The listing builds one solid part. Answer for the finished solid, in the listing's coordinates (mm). A direction names the side the tool comes from. Give positions to 0.01 mm unless a question says otherwise; leave off trailing zeros. Loops run counter-clockwise (first coordinate to the right, second up) from the corner with the lowest first, then second, coordinate; pieces in that order, holes last. Notation, with made-up numbers: (20.5, 69) - (44.5, 69) arc R24 cw to (44.5, 105) - close; hole circle Ø1 at (80, 6.5). An arc over 180 degrees is marked (long way). Write each question's results on one line, items separated by ' | '.
Autodesk Inventor part; units mm, degrees
ref_plane "YZ Plane" through (0, 0, 0) normal (1, 0, 0) x (0, 1, 0)
ref_plane "XZ Plane" through (0, 0, 0) normal (0, 1, 0) x (-1, 0, 0)
ref_plane "XY Plane" through (0, 0, 0) normal (0, 0, 1) x (1, 0, 0)
sketch "Skizze1" plane through (0, 0, 0) normal (0, 0, 1) x (1, 0, 0)
  line L0 (-20, -3.5) -> (20, -3.5)
  line L1 (20, -3.5) -> (20, 3.5)
  line L2 (20, 3.5) -> (-20, 3.5)
  line L3 (-20, 3.5) -> (-20, -3.5)
  line L4 (-20, -3.5) -> (20, 3.5) construction
  line L5 (20, -3.5) -> (-20, 3.5) construction
  line L6 (3.5, -20) -> (-3.5, -20)
  line L7 (-3.5, -20) -> (-3.5, 20)
  line L8 (-3.5, 20) -> (3.5, 20)
  line L9 (3.5, 20) -> (3.5, -20)
  line L10 (3.5, -20) -> (-3.5, 20) construction
  line L11 (-3.5, -20) -> (3.5, 20) construction
  point P0 (0, 0)
  dimension "d0" = 7
  dimension "d1" = 40
extrude "Extrusion1" add sketch "Skizze1" along normal blind 1.5
fillet "Rundung1" radius 3.5 8 edges at (3.5, 20, 0.75) (-3.5, 20, 0.75) (20, 3.5, 0.75) (20, -3.5, 0.75) (3.5, -20, 0.75) (-3.5, -20, 0.75) (-20, -3.5, 0.75) (-20, 3.5, 0.75)
fillet "Rundung2" radius 6 4 edges at (3.5, 3.5, 0.75) (-3.5, 3.5, 0.75) (-3.5, -3.5, 0.75) (3.5, -3.5, 0.75)
sketch "Skizze2" plane through (0, 0, 1.5) normal (0, 0, 1) x (1, 0, 0)
  circle A0 centre (0, 0) radius 5
  circle A1 centre (16.5, 0) radius 1.6
  circle A2 centre (-16.5, 0) radius 1.6
  circle A3 centre (0, 16.5) radius 1.6
  circle A4 centre (0, -16.5) radius 1.6
  circle A5 centre (0, -8) radius 1.6
  circle A6 centre (0, 8) radius 1.6
  circle A7 centre (-9.5, 0) radius 1.6
  circle A8 centre (9.5, 0) radius 1.6
  line L0 (0, 16.5) -> (0, -16.5) construction
  line L1 (-16.5, 0) -> (16.5, 0) construction
  line L2 (9.5, 0) -> (-9.5, 0) construction
  line L3 (0, 8) -> (0, -8) construction
  dimension "d6" = 3.2
  dimension "d7" = 10
  dimension "d8" = 33
  dimension "d9" = 19
  dimension "d10" = 16
extrude "Extrusion2" cut sketch "Skizze2" against normal blind 1.5
chamfer "Fase1" distance 0.7 angle 45 4 edges at (-1.6, -8, 1.5) (-11.1, 0, 1.5) (-1.6, 8, 1.5) (7.9, 0, 1.5)
chamfer "Fase2" distance 0.7 angle 45 4 edges at (-1.6, 16.5, 0) (-18.1, 0, 0) (-1.6, -16.5, 0) (14.9, 0, 0)
equation "\"G_L\" = 0"
equation "\"G_H\" = 0"
equation "\"G_B\" = 0"
properties part number "Motorkreuz_klein" material "GEDA Stahl"
Item 1: For faces 4 (the face through (3.5, 13, 1)), 5 (the face through (3.5, -13, 1)), 6 (the face through (-19, -2.45, 0.76)), determine the directions among +Z, -Z, +X, -X, +Y, -Y from which every point of the face is accessible in a straight line to the end or side of a thin tool.
Values found:
face 4: +Z, -Z, +X, +Y | face 5: +Z, -Z, +X, -Y | face 6: +Z, -Z, -X, -Y
Item 2: A cutting plane is placed at A-A, the plane z = 0.45. Count the separate pieces of the cut face and the enclosed holes in it, plus the area to 3 significant figures.
Values found:
separate pieces: 1 | enclosed holes: 9 | area: 367 mm²
Item 3: Flat-ended cylindrical pins translate along their axes: P1, Ø5, axis at x = -9.5, y = 0, coming from the -Z side; P2, Ø0.8, axis at y = -13, z = 0.5, coming from the +X side; P3, Ø3.5, axis at x = 0, y = 16.5, coming from the -Z side. Find the tip coordinate at first contact, or state that the pin passes through.
Values found:
P1: stops at z = 0 | P2: stops at x = 3.5 | P3: stops at z = 0.55
Item 4: A cutting plane is placed at B-B, the plane x = 4. Determine the outline of the cut face in (y, z).
Values found:
outline: (-7.1, 0) - (-3, 0) - (-3, 1.5) - (-7.1, 1.5) - close; (3, 0) - (7.1, 0) - (7.1, 1.5) - (3, 1.5) - close
Item 5: Find the intervals of material crossed by line 1 along X through (y, z) = (-1, 0.3); line 2 along Y through (x, z) = (9.5, 0.4); line 3 along X through (y, z) = (1, 0.55), in increasing order. Write a range as [from, to].
Values found:
line 1: x = [-19.85, -18.23], [-14.77, -10.75], [-8.25, -4.9], [4.9, 8.25], [10.75, 14.77], [18.23, 19.85] | line 2: y = [-3.5, -1.6], [1.6, 3.5] | line 3: x = [-19.85, -17.94], [-15.06, -10.75], [-8.25, -4.9], [4.9, 8.25], [10.75, 15.06], [17.94, 19.85]
Item 6: For a pull along Y with two mould halves and no side action, classify faces 1 (the face through (-0.35, 6.44, 0.41)), 2 (the face through (-3.5, -13, 1)), 3 (the face through (-2.45, 19, 0.76)) as released by +Y, released by -Y, zero draft, split by the parting line, or undercut.
Values found:
face 1: undercut | face 2: zero draft | face 3: released by +Y
Item 7: A cutting plane is placed at D-D, the plane y = 8. Determine the outline of the cut face in (x, z), plus the area to 3 significant figures.
Values found:
outline: (-3.69, 0) - (-1.6, 0) - (-1.6, 0.8) - (-2.3, 1.5) - (-3.69, 1.5) - close; (1.6, 0) - (3.69, 0) - (3.69, 1.5) - (2.3, 1.5) - (1.6, 0.8) - close | area: 5.78 mm²
